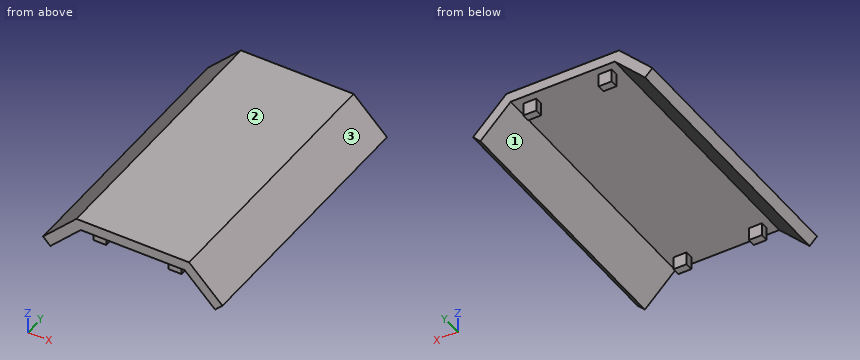
```python
from build123d import *

# Parameters (mm, degrees)
SALIENTE_EXTRUIR1_DEPTH = 103
CROQUIS2_W              = 10
CROQUIS2_H              = 6
SALIENTE_EXTRUIR2_DEPTH = 10


with BuildPart() as part:
    # Croquis1 → Saliente-Extruir1 (new, symmetric)
    with BuildSketch(Plane(origin=(0, 0, 0), x_dir=(1, 0, 0), z_dir=(0, 1, 0))):
        Polygon((-40, 0), (40, 0), (63.334523779, 23.334523779), (68.991378029, 17.67766953), (43.313708499, -8), (-43.313708499, -8), (-68.991378029, 17.67766953), (-63.334523779, 23.334523779), align=None)
    extrude(amount=SALIENTE_EXTRUIR1_DEPTH, both=True)

    # Croquis2 → Saliente-Extruir2 (add)
    with BuildSketch(Plane(origin=(0, 0, 0), x_dir=(-1, 0, 0), z_dir=(0, 0, -1))):
        with Locations((29, -94)):
            Rectangle(CROQUIS2_W, CROQUIS2_H)
        with Locations((-29, -94)):
            Rectangle(CROQUIS2_W, CROQUIS2_H)
    saliente_extruir2 = extrude(amount=SALIENTE_EXTRUIR2_DEPTH)

    # Simetría2: Saliente-Extruir2 across plane
    add(saliente_extruir2.mirror(Plane.ZX))


solid = part.part
```
For this review, take the finished solid that the model builds, in its own axes (mm). Face numbers are marked on the shaded views. Round coordinates to 2 decimals unless told otherwise and drop trailing zeros. Write each loop counter-clockwise with the first axis right and the second up, starting at its lowest first coordinate (ties: lowest second). Pieces come first, ordered by that corner, then holes.
1) Insertion check: pin 1 Ø6.5 at (y, z) = (95, -3.5) entering from +X; pin 2 Ø11 at (x, z) = (-27, -7.5) entering from -Y; pin 3 Ø8 at (x, z) = (26.5, -3) entering from +Y; pin 4 Ø6.5 at (y, z) = (94, -4) entering from +X. Each pin has a flat end and moves straight along its axis. Give the tip position at first contact, or say it passes through.
Answer below:
pin 1: stops at x = 58.06
pin 2: stops at y = -97
pin 3: stops at y = 103
pin 4: stops at x = 58.56
2) For line 1 along Z through (x, y) = (40, 77); line 2 along X through (y, z) = (-61.5, -17); line 3 along X through (y, z) = (49.5, -20), list the stretches that pass through material, from the lowest coordinate up.
Answer below:
line 1: z = 0 to 8
line 2: x = -68.31 to -57, 57 to 68.31
line 3: x = -66.67 to -60, 60 to 66.67
3) Take a section at B-B on y = 86.5. Give the boundary of the cut face in (x, z), then the cut area to 3 significant figures.
Answer below:
outline: (-68.99, -17.68) - (-63.33, -23.33) - (-40, 0) - (40, 0) - (63.33, -23.33) - (68.99, -17.68) - (43.31, 8) - (-43.31, 8) - close
area: 1,220 mm2
4) Take a section at D-D on x = 10. Give the boundary of the cut face in (y, z).
Answer below:
outline: (-103, 0) - (103, 0) - (103, 8) - (-103, 8) - close
5) Mouldability with a two-part tool opening along X and no side actions: class the marked faces 1, 2 and 3 as +X half, -X half, draft (parallel to the pull), parting line (faces both ways), or undercut.
Answer below:
face 1: undercut
face 2: draft
face 3: +X half
6) Take a section at C-C on z = -5.5. Give the boundary of the cut face in (x, y), then the cut area to 3 significant figures.
Answer below:
outline: (-56.81, -103) - (-45.5, -103) - (-45.5, 103) - (-56.81, 103) - close; (-34, -97) - (-24, -97) - (-24, -91) - (-34, -91) - close; (-34, 91) - (-24, 91) - (-24, 97) - (-34, 97) - close; (24, -97) - (34, -97) - (34, -91) - (24, -91) - close; (24, 91) - (34, 91) - (34, 97) - (24, 97) - close; (45.5, -103) - (56.81, -103) - (56.81, 103) - (45.5, 103) - close
area: 4,900 mm2
7) Take a section at A-A on z = -15. Give the boundary of the cut face in (x, y), then the cut area to 3 significant figures.
Answer below:
outline: (-66.31, -103) - (-55, -103) - (-55, 103) - (-66.31, 103) - close; (55, -103) - (66.31, -103) - (66.31, 103) - (55, 103) - close
area: 4,660 mm2
